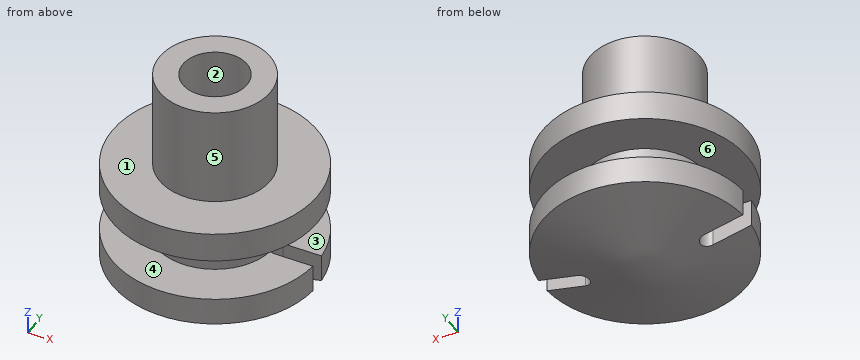
```python
from build123d import *

# Parameters (mm, degrees)
SKETCH1_R           = 9.25
BOSS_EXTRUDE1_DEPTH = 2.5
SKETCH2_R           = 5.35
BOSS_EXTRUDE2_DEPTH = 3.9
SKETCH3_R           = 9.25
BOSS_EXTRUDE3_DEPTH = 2.7
SKETCH4_R           = 5
BOSS_EXTRUDE4_DEPTH = 9
CUT_EXTRUDE1_DEPTH  = 4.5
SKETCH8_R           = 2.9
CUT_EXTRUDE2_DEPTH  = 12


with BuildPart() as part:
    # Sketch1 → Boss-Extrude1 (new body)
    with BuildSketch(Plane.XY):
        Circle(SKETCH1_R)
    extrude(amount=BOSS_EXTRUDE1_DEPTH)

    # Sketch2 → Boss-Extrude2 (add)
    with BuildSketch(Plane.XY.offset(2.5)):
        Circle(SKETCH2_R)
    extrude(amount=BOSS_EXTRUDE2_DEPTH)

    # Sketch3 → Boss-Extrude3 (add)
    with BuildSketch(Plane.XY.offset(6.4)):
        Circle(SKETCH3_R)
    extrude(amount=BOSS_EXTRUDE3_DEPTH)

    # Sketch4 → Boss-Extrude4 (add)
    with BuildSketch(Plane.XY.offset(9.1)):
        Circle(SKETCH4_R)
    extrude(amount=BOSS_EXTRUDE4_DEPTH)

    # Sketch6 → Revolve1 (revolve)
    with BuildSketch(Plane(origin=(0, 0, 0), x_dir=(1, 0, 0), z_dir=(0, 1, 0)), mode=Mode.PRIVATE) as revolve1_sk:
        Polygon((0, 0), (0, 2), (9.25, 0), align=None)
    revolve(revolve1_sk.sketch.rotate(Axis((0, 0, 0), (0, 0, -1)), 180), axis=Axis((0, 0, 0), (0, 0, -1)))

    # Sketch7 → Cut-Extrude1 (cut, symmetric)
    with BuildSketch(Plane.XY):
        with BuildLine():
            Line((-5.75, 0.75), (-9.219544457, 0.75))
            ThreePointArc((-9.219544457, 0.75), (-9.25, 0), (-9.219544457, -0.75))
            Line((-9.219544457, -0.75), (-5.75, -0.75))
            ThreePointArc((-5.75, -0.75), (-5, 0), (-5.75, 0.75))
        make_face()
        with BuildLine():
            Line((5.75, -0.75), (9.219544457, -0.75))
            ThreePointArc((9.219544457, -0.75), (9.25, 0), (9.219544457, 0.75))
            Line((9.219544457, 0.75), (5.75, 0.75))
            ThreePointArc((5.75, 0.75), (5, 0), (5.75, -0.75))
        make_face()
    extrude(amount=CUT_EXTRUDE1_DEPTH, both=True, mode=Mode.SUBTRACT)

    # Sketch8 → Cut-Extrude2 (cut)
    with BuildSketch(Plane.XY.offset(18.1)):
        Circle(SKETCH8_R)
    extrude(amount=-CUT_EXTRUDE2_DEPTH, mode=Mode.SUBTRACT)


solid = part.part
```
Read the model definition and answer for the solid it produces. Units are mm, in the model's axes. Face numbers are marked on the shaded views. A direction names the side the tool comes from. Give positions to 0.01 mm unless a question says otherwise; leave off trailing zeros. Write each loop counter-clockwise with the first axis right and the second up, starting at its lowest first coordinate (ties: lowest second). Pieces come first, ordered by that corner, then holes. Notation, with made-up numbers: M 39,56.5 L 68,56.5 A23 cw 68,75.5 Z; hole C -23,-37 d7. An arc over 180 degrees is marked long. Put each result on its own line as item: value. Start each with the question number.
1. Each of these flat-tipped pins is pushed along its axis until it touches: pin 1 Ø4 at (x, z) = (6.5, 6.5) entering from -Y; pin 2 Ø1 at (x, z) = (-6.5, 0.5) entering from +Y; pin 3 Ø3.5 at (x, z) = (8, 1.5) entering from -Y; pin 4 Ø6.5 at (x, y) = (0, 0) entering from +Z. Where does it stop, or does it pass through?
2. Which of the six approach directions +Z, -Z, +X, -X, +Y, -Y give full straight-line access (tool end or side, diameter ignored) to the marked faces 4, 5 and 6?
3. The part is cut by section C-C, the plane x = -7.75. Give the number of separate pieces and of enclosed holes in the cut face, and give its area (3 significant figures).
4. For a pull along Z with two mould halves and no side action, classify the marked faces 1, 2 and 3 as released by +Z, released by -Z, zero draft, split by the parting line, or undercut.
5. The part is cut by section D-D, the plane z = 7. Give the vertices of the cut face in (x, y).
6. Consider line 1 along Y through (x, z) = (0, 13.75); line 2 along Z through (x, y) = (-7.75, 5); line 3 along X through (y, z) = (-0.25, 6). Determine where each line is inside the solid, lowest interval first.
7. The part is cut by section B-B, the plane z = 12.5. Give the vertices of the cut face in (x, y), and give its area (3 significant figures).
8. The part is cut by section A-A, the plane z = 1.5. Give the vertices of the cut face in (x, y), and give its area (3 significant figures).
Final values:
1. pin 1: stops at y = -8.08
1. pin 2: stops at y = 7.04
1. pin 3: stops at y = -6.82
1. pin 4: stops at z = 18.1
2. face 4: -Y
2. face 5: +Z
2. face 6: none
3. separate pieces: 3
3. enclosed holes: 0
3. area: 50.4 mm²
4. face 1: released by +Z
4. face 2: zero draft
4. face 3: undercut
5. outline: C 0,0 d18.5; hole C 0,0 d5.8
6. line 1: y = -5 to -2.9, 2.9 to 5
6. line 2: z = -0.01 to 2.5, 6.4 to 9.1
6. line 3: x = -5.34 to 5.34
7. outline: C 0,0 d10; hole C 0,0 d5.8
7. area: 52.1 mm²
8. outline: M -9.22,-0.75 A9.25 ccw 9.22,-0.75 L 5.75,-0.75 A0.75 cw 5.75,0.75 L 9.22,0.75 A9.25 ccw -9.22,0.75 L -5.75,0.75 A0.75 cw -5.75,-0.75 Z
8. area: 257 mm²
